Can you work these out from the drawing? Everything is in mm from the part's minimum corner. A direction names the side the tool comes from. Round coordinates to 2 decimals unless told otherwise and drop trailing zeros. Loops run counter-clockwise (first coordinate to the right, second up) from the corner with the lowest first, then second, coordinate; pieces in that order, holes last. Notation, with made-up numbers: (73.25, 63) - (86.25, 63) arc R26 ccw to (86.25, 86) - close; hole circle Ø8 at (30.25, -23.75). An arc over 180 degrees is marked (long way). Answer as a JSON object with one key per item and string values. Group by question number.
1) I want a section at A-A, the plane z = 7. Please give me the cut outline in (x, y), then the cut area to 3 significant figures.
2) I want a section at C-C, the plane x = 9. Please give me the cut outline in (y, z), then the cut area to 3 significant figures.
3) I want a section at D-D, the plane x = 17.5. Please give me the cut outline in (y, z), then the cut area to 3 significant figures.
4) Which directions (+Z, -Z, +X, -X, +Y, -Y) give clear straight access to the entire face, cutting with the end or side of a thin tool? Please do the marked faces 1 and 2.
5) If I drill on line 1 along Y through (x, z) = (3.5, 7); line 2 along X through (y, z) = (10.25, 1); line 3 along Y through (x, z) = (9, 10.5), over which ranges is the centre line in solid material (lowest first)? Write a range as [from, to].
6) Will these pins go through, and if not, where does the flat tip stop? P1, Ø5, axis at x = 16.5, z = 2.5, coming from the +Y side; P2, Ø8, axis at x = 9.5, y = 11.5, coming from the +Z side.
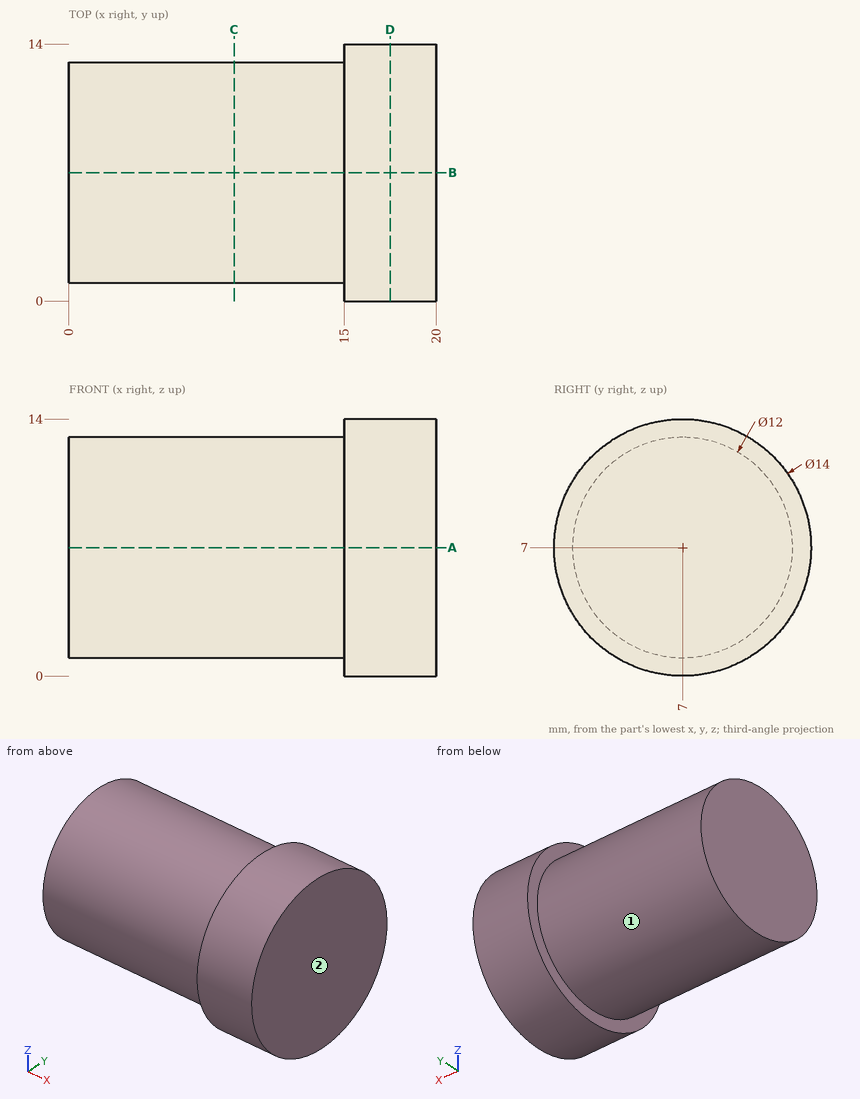
Outcome:
{
 "1": {"outline": "(0, 1) - (15, 1) - (15, 0) - (20, 0) - (20, 14) - (15, 14) - (15, 13) - (0, 13) - close", "area": "250 mm^2"},
 "2": {"outline": "circle Ø12 at (7, 7)", "area": "113 mm^2"},
 "3": {"outline": "circle Ø14 at (7, 7)", "area": "154 mm^2"},
 "4": {"face 1": "-X", "face 2": "+Z, -Z, +X, +Y, -Y"},
 "5": {"line 1": "[1, 13]", "line 2": "[15, 20]", "line 3": "[2.13, 11.87]"},
 "6": {"P1": "y = 13.71", "P2": "z = 12.98"}
}
